```python
from build123d import *

# Parameters (mm, degrees)
ESBO_O1_R                = 7
ESBO_O1_R_2              = 3
RESSALTO_EXTRUS_O1_DEPTH = 1.8
ESBO_O2_R                = 6.25
RESSALTO_EXTRUS_O2_DEPTH = 11
CORTE_EXTRUS_O1_START    = -11
ESBO_O3_R                = 3
CORTE_EXTRUS_O1_DEPTH    = 11
ESBO_O4_R                = 0.5
RESSALTO_EXTRUS_O3_DEPTH = 9
FILETE1_R                = 0.5
ESBO_O5_W                = 4
ESBO_O5_H                = 0.265788673
ESBO_O5_W_2              = 0.206724524
ESBO_O5_H_2              = 4
RESSALTO_EXTRUS_O4_DEPTH = 4.5
CORTE_EXTRUS_O2_DEPTH    = 2.25
CORTE_EXTRUS_O3_DEPTH    = 2.25


with BuildPart() as part:
    # Esboço1 → Ressalto-extrusão1 (new body)
    with BuildSketch(Plane.XY):
        Circle(ESBO_O1_R)
        with Locations((0, 3)):
            Circle(ESBO_O1_R_2, mode=Mode.SUBTRACT)
    extrude(amount=RESSALTO_EXTRUS_O1_DEPTH)

    # Esboço2 → Ressalto-extrusão2 (add)
    with BuildSketch(Plane(origin=(0, 0, 0), x_dir=(-1, 0, 0), z_dir=(0, 0, -1))):
        with Locations(Location((0, 0, 0), (0, 0, 180))):
            Circle(ESBO_O2_R)
    extrude(amount=RESSALTO_EXTRUS_O2_DEPTH)

    # Esboço3 → Corte-extrusão1 (cut)
    with BuildSketch(Plane.XY.offset(1.8).offset(CORTE_EXTRUS_O1_START)):
        with Locations((0, 3)):
            Circle(ESBO_O3_R)
    extrude(amount=CORTE_EXTRUS_O1_DEPTH, mode=Mode.SUBTRACT)

    # Esboço4 → Ressalto-extrusão3 (add)
    with BuildSketch(Plane.XY.offset(-9.2)):
        with Locations((0, 3)):
            Circle(ESBO_O4_R)
    extrude(amount=RESSALTO_EXTRUS_O3_DEPTH)

    # Filete1
    filete1_edges = [part.edges().sort_by_distance(p)[0] for p in [
        (-0.5, 3, -0.2),
    ]]
    fillet(filete1_edges, radius=FILETE1_R)

    # Esboço5 → Ressalto-extrusão4 (add)
    with BuildSketch(Plane(origin=(0, 0, -11), x_dir=(-1, 0, 0), z_dir=(0, 0, -1))):
        with Locations((0.095181179, -5.212411193)):
            Rectangle(ESBO_O5_W, ESBO_O5_H)
        with Locations((5.289644951, -0.001979347)):
            Rectangle(ESBO_O5_W_2, ESBO_O5_H_2)
    extrude(amount=RESSALTO_EXTRUS_O4_DEPTH)

    # Esboço6 → Corte-extrusão2 (cut, symmetric)
    with BuildSketch(Plane.ZY.offset(5.393007213)):
        with BuildLine():
            Line((-15.5, -2.001979347), (-14, -2.001979347))
            ThreePointArc((-14, -2.001979347), (-15.060660172, -1.562639519), (-15.5, -0.501979347))
            Line((-15.5, -0.501979347), (-15.5, -2.001979347))
        make_face()
        with BuildLine():
            Line((-15.5, 1.998020653), (-15.5, 0.498020653))
            ThreePointArc((-15.5, 0.498020653), (-15.060660172, 1.558680825), (-14, 1.998020653))
            Line((-14, 1.998020653), (-15.5, 1.998020653))
        make_face()
    extrude(amount=CORTE_EXTRUS_O2_DEPTH, both=True, mode=Mode.SUBTRACT)

    # Esboço7 → Corte-extrusão3 (cut, symmetric)
    with BuildSketch(Plane.XZ.offset(5.345305529)):
        with BuildLine():
            Line((1.904818821, -15.5), (1.904818821, -14))
            ThreePointArc((1.904818821, -14), (1.465478993, -15.060660172), (0.404818821, -15.5))
            Line((0.404818821, -15.5), (1.904818821, -15.5))
        make_face()
        with BuildLine():
            Line((-2.095181179, -15.5), (-0.595181179, -15.5))
            ThreePointArc((-0.595181179, -15.5), (-1.655841351, -15.060660172), (-2.095181179, -14))
            Line((-2.095181179, -14), (-2.095181179, -15.5))
        make_face()
    extrude(amount=CORTE_EXTRUS_O3_DEPTH, both=True, mode=Mode.SUBTRACT)


solid = part.part
```
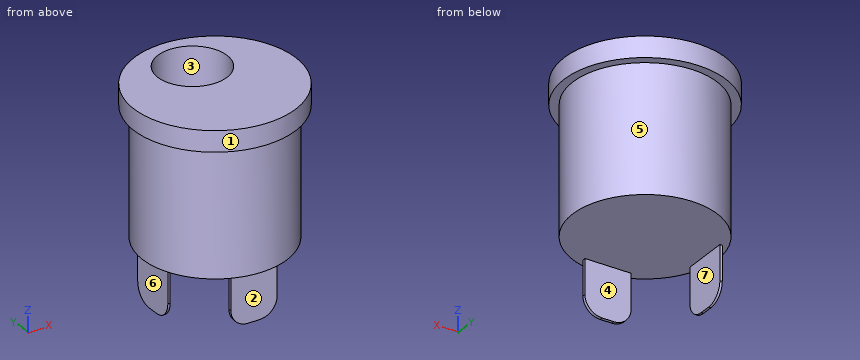
Input: part model. Units: mm. Frame: model coordinates. Face numbers are marked on the shaded views. A direction names the side the tool comes from. Round coordinates to 2 decimals unless told otherwise and drop trailing zeros. Order: outer loops, then holes, each group sorted by start corner. A loop starts at its lowest first (then second) coordinate and runs counter-clockwise, first axis right, second up. Notation, with made-up numbers: (-10, -10.5) - (26, -10.5) arc R27 ccw to (26, 16.5) - close; hole circle Ø10 at (33, -2.75). An arc over 180 degrees is marked (long way). One line per question, with ' | ' between items. Start each with the question number.
1) Pull-direction query (X, two-part tool) for the marked faces 1, 2 and 3; classes: +X half, -X half, draft (parallel to the pull), parting line (faces both ways), or undercut.
2) Cut plane B-B, the plane x = 0. Return the cut outline in (y, z).
3) Cut plane D-D, the plane z = 0.25. Return the cut outline in (x, y).
4) Cut plane A-A, the plane z = -13.75. Return the cut outline in (x, y).
5) Cut plane C-C, the plane y = -4.5. Return the cut outline in (x, z).
6) Ray query, probe 1 along Y at (x, z) = (0, -2.75); probe 2 along Z at (x, y) = (-1, 6); probe 3 along Z at (x, y) = (-1, 6.25). Return the intervals inside material, ascending.
7) Contact query for flat-ended pins moving along their axis: P1, Ø5.5, axis at x = 0, y = 3, coming from the -Z side; P2, Ø1.2, axis at y = -0.5, z = -13.5, coming from the -X side; P3, Ø1, axis at x = -2.5, z = -3.5, coming from the -Y side. Output: stop coordinate, or through.
8) Set-up query: the marked faces 4, 5, 6 and 7. Return all of +Z, -Z, +X, -X, +Y, -Y with unobstructed straight access to the full face (end or side cutting, diameter ignored); none if empty.
Worked out:
1) face 1: parting line | face 2: draft | face 3: undercut
2) outline: (-7, 0) - (-6.25, 0) - (-6.25, -11) - (-5.35, -11) - (-5.35, -15.5) - (-5.08, -15.5) - (-5.08, -11) - (6.25, -11) - (6.25, 0) - (7, 0) - (7, 1.8) - (6, 1.8) - (6, -9.2) - (3.5, -9.2) - (3.5, -0.7) arc R0.5 ccw to (2.5, -0.7) - (2.5, -9.2) - (0, -9.2) - (0, 1.8) - (-7, 1.8) - close
3) outline: circle Ø14 at (0, 0); hole circle Ø6 at (0, 3)
4) outline: (-5.39, -2) - (-5.19, -2) - (-5.19, 2) - (-5.39, 2) - close; (-2.1, -5.35) - (1.9, -5.35) - (1.9, -5.08) - (-2.1, -5.08) - close
5) outline: (-5.36, 0) - (-4.34, 0) - (-4.34, -11) - (4.34, -11) - (4.34, 0) - (5.36, 0) - (5.36, 1.8) - (-5.36, 1.8) - close
6) probe 1: y = -6.25 to 0, 2.5 to 3.5, 6 to 6.25 | probe 2: z = -11 to 1.8 | probe 3: z = 0 to 1.8
7) P1: stops at z = -11 | P2: stops at x = -5.39 | P3: stops at y = -5.92
8) face 4: -Z, +X, -X, +Y | face 5: -Z | face 6: -Z, -X, +Y, -Y | face 7: -Z, +X, +Y, -Y
